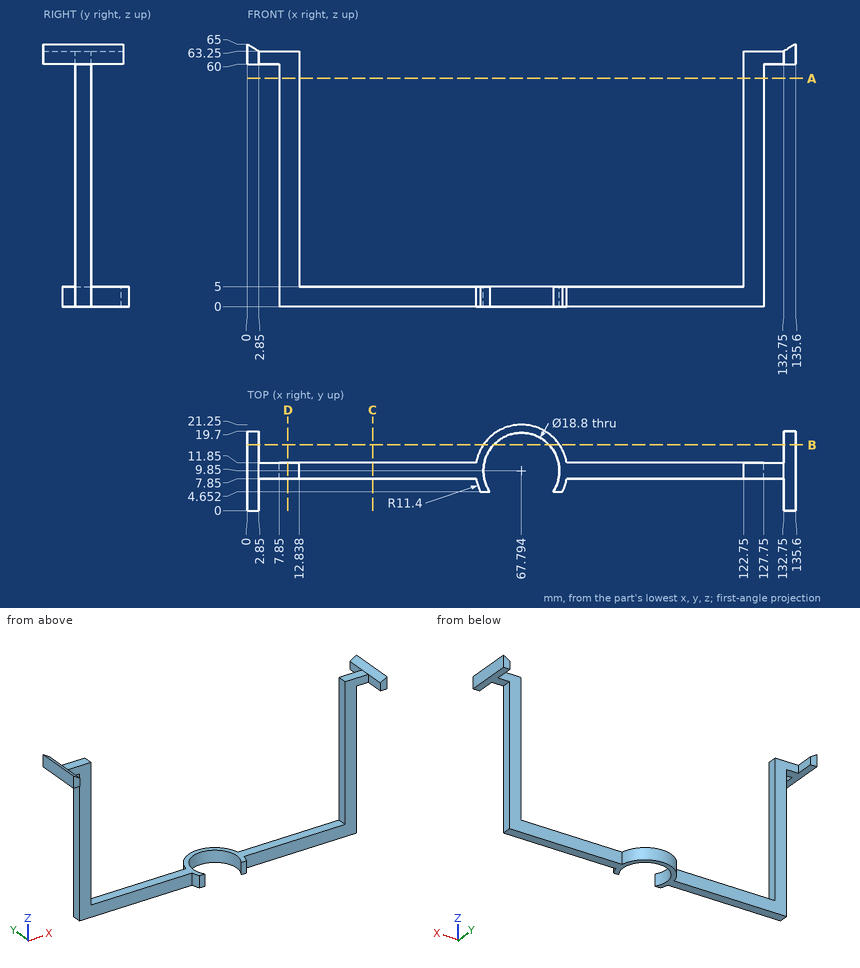
The figure shows three views and two pictorial views of one solid part (mm, origin at its lowest corner). Answer the questions. Give positions to 0.01 mm unless a question says otherwise; leave off trailing zeros. Write each loop counter-clockwise with the first axis right and the second up, starting at its lowest first coordinate (ties: lowest second). Pieces come first, ordered by that corner, then holes.
Q1. The part is cut by section D-D on x = 10. Give the vertices of the cut face in (y, z).
Answer:
outline: (7.85, 0) - (11.85, 0) - (11.85, 63.25) - (7.85, 63.25) - close
Q2. The part is cut by section A-A on z = 56.5. Give the vertices of the cut face in (x, y).
Answer:
outline: (7.85, 7.85) - (12.84, 7.85) - (12.84, 11.85) - (7.85, 11.85) - close; (122.75, 7.85) - (127.75, 7.85) - (127.75, 11.85) - (122.75, 11.85) - close
Q3. Given pin 1 (12 mm diameter, centred on x = 24.5, z = 49, fed in from -Y); pin 2 (4 mm diameter, centred on y = 10, z = 34.5, fed in from +X); pin 3 (2.5 mm diameter, centred on x = 134.5, z = 63, fed in from +Y); pin 4 (8.5 mm diameter, centred on x = 2.5, y = 11, fed in from -Z), each flat-ended and moving along its own axis, determine where each tip first touches the part or whether it passes through.
Answer:
pin 1: passes through
pin 2: stops at x = 127.75
pin 3: stops at y = 19.7
pin 4: stops at z = 60
Q4. Straight lines are drawn through the part: L1, parallel to X at y = 8.75, z = 53.5; L2, parallel to X at y = 10.5, z = 4; L3, parallel to Z at x = 115, y = 10.75. For each, find the intervals that lie inside material, in ascending order.
Answer:
L1: x = 7.85 to 12.84, 122.75 to 127.75
L2: x = 7.85 to 58.42, 77.17 to 127.75
L3: z = 0 to 5
Q5. The part is cut by section B-B on y = 16.25. Give the vertices of the cut face in (x, z).
Answer:
outline: (0, 60) - (2.85, 60) - (2.85, 63.25) - (0, 65) - close; (58.36, 0) - (60.91, 0) - (60.91, 5) - (58.36, 5) - close; (74.68, 0) - (77.23, 0) - (77.23, 5) - (74.68, 5) - close; (132.75, 60) - (135.6, 60) - (135.6, 65) - (132.75, 63.25) - close
Q6. The part is cut by section C-C on x = 31. Give the vertices of the cut face in (y, z).
Answer:
outline: (7.85, 0) - (11.85, 0) - (11.85, 5) - (7.85, 5) - close
